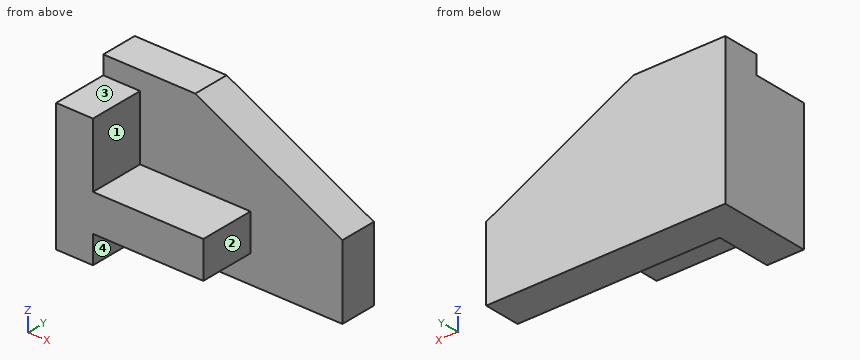
from build123d import *

# Parameters (mm, degrees)
F1_DEPTH = 25
F2_DEPTH = 10
F0_W     = 30
F0_H     = 10
F3_DEPTH = 25


with BuildPart() as f1:
    # F0 (on Front) → F1 (new body)
    with BuildSketch(Plane.XZ):
        Polygon((-64.929679, 35.287431), (-74.929679, 35.287431), (-74.929679, 0.287431), (-64.929679, 0.287431), (-64.929679, 7.787431), (-64.929679, 17.787431), align=None)
    extrude(amount=F1_DEPTH)

    # F0 (on Front) → F2 (join)
    with BuildSketch(Plane.XZ):
        Polygon((-74.929679, 40.287431), (-74.929679, 35.287431), (-64.929679, 35.287431), (-64.929679, 17.787431), (-34.929679, 17.787431), (-34.929679, 7.787431), (-64.929679, 7.787431), (-64.929679, 0.287431), (-9.929679, 0.287431), (-9.929679, 20.287431), (-49.929679, 40.287431), align=None)
    extrude(amount=F2_DEPTH)

    # F0 (on Front) → F3 (join)
    with BuildSketch(Plane.XZ):
        with Locations((-49.929679, 12.787431)):
            Rectangle(F0_W, F0_H)
    extrude(amount=F3_DEPTH)


solid = f1.part
Design review of the part built by this model. Coordinates are the model's own, in mm. Face numbers are marked on the shaded views. A direction names the side the tool comes from. Coordinates: 2 decimals unless noted, no trailing zeros. Write each loop counter-clockwise with the first axis right and the second up, starting at its lowest first coordinate (ties: lowest second). Pieces come first, ordered by that corner, then holes. Notation, with made-up numbers: (77.25, 75.5) - (85.25, 75.5) arc R27 cw to (85.25, 111.5) - close; hole circle Ø11 at (73, -15). An arc over 180 degrees is marked (long way). Use one line per item in the form item = value.
Q1. Consider section D-D (x = -69). Write out the cut boundary in (y, z).
Taken from the geometry:
outline = (-25, 0.29) - (0, 0.29) - (0, 40.29) - (-10, 40.29) - (-10, 35.29) - (-25, 35.29) - close
Q2. Consider section C-C (z = 6.5). Write out the cut boundary in (x, y), plus the area to 3 significant figures.
Taken from the geometry:
outline = (-74.93, -25) - (-64.93, -25) - (-64.93, -10) - (-9.93, -10) - (-9.93, 0) - (-74.93, 0) - close
area = 800 mm^2
Q3. Insertion check: pin 1 Ø2 at (y, z) = (-15, 3) entering from +X; pin 2 Ø8 at (x, y) = (-68.5, -20) entering from +Z. Each pin has a flat end and moves straight along its axis. Give the tip position at first contact, or say it passes through.
Taken from the geometry:
pin_1 = -64.93
pin_2 = 35.29
Q4. Consider section B-B (y = -20.5). Write out the cut boundary in (x, z).
Taken from the geometry:
outline = (-74.93, 0.29) - (-64.93, 0.29) - (-64.93, 7.79) - (-34.93, 7.79) - (-34.93, 17.79) - (-64.93, 17.79) - (-64.93, 35.29) - (-74.93, 35.29) - close
Q5. Machinability: for the marked faces 1, 2, 3 and 4, which of the approach directions +Z, -Z, +X, -X, +Y, -Y give a long, thin tool a straight path to every point of the face, cutting with its end or side? Answer none if there is none.
Taken from the geometry:
face_1 = +Z, +X, -Y
face_2 = +Z, -Z, +X, -Y
face_3 = +Z, +X, -X, -Y
face_4 = -Z, +X, -Y
Q6. Consider section A-A (x = -56.5). Write out the cut boundary in (y, z), plus the area to 3 significant figures.
Taken from the geometry:
outline = (-25, 7.79) - (-10, 7.79) - (-10, 0.29) - (0, 0.29) - (0, 40.29) - (-10, 40.29) - (-10, 17.79) - (-25, 17.79) - close
area = 550 mm^2
Q7. For probe 1 along Y at (x, z) = (-55, 25.5); probe 2 along X at (y, z) = (-21.5, 17); probe 3 along Z at (x, y) = (-67.5, -12.25), list the stretches that pass through material, from the lowest coordinate up.
Taken from the geometry:
probe_1 = -10 to 0
probe_2 = -74.93 to -34.93
probe_3 = 0.29 to 35.29
